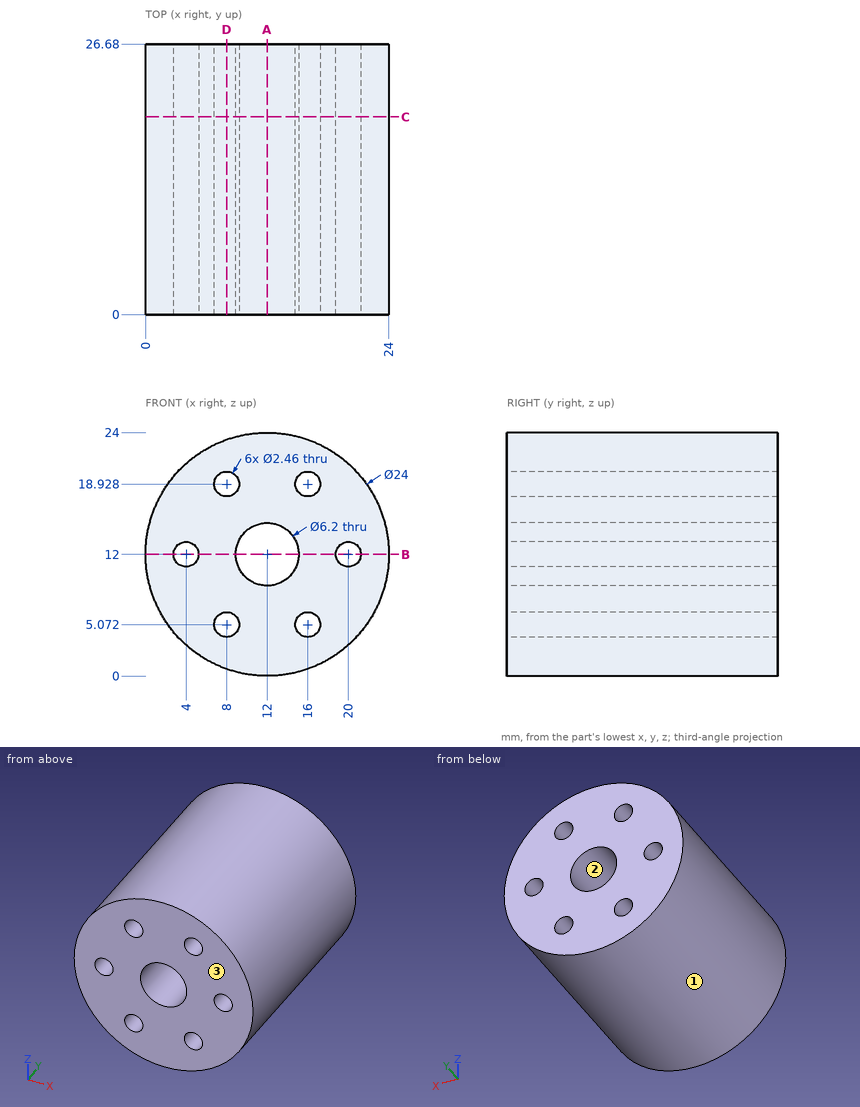
Geometry: see drawing. Coordinates: mm, zero at the bounding-box minimum. Give positions to 0.01 mm unless a question says otherwise; leave off trailing zeros. Order: outer loops, then holes, each group sorted by start corner. A loop starts at its lowest first (then second) coordinate and runs counter-clockwise, first axis right, second up. Notation, with made-up numbers: (77, -11.75) -> (99, -11.75) arc R14 cw to (99, -1.75) -> close; hole circle Ø9 at (-37.5, 75). An arc over 180 degrees is marked (long way). Write each question's results on one line, items separated by ' | '.
1) Cut plane D-D (x = 8). Output: boundary loops of the cut face in (y, z).
Geometry says:
outline: (0, 0.69) -> (26.68, 0.69) -> (26.68, 3.84) -> (0, 3.84) -> close; (0, 6.3) -> (26.68, 6.3) -> (26.68, 17.7) -> (0, 17.7) -> close; (0, 20.16) -> (26.68, 20.16) -> (26.68, 23.31) -> (0, 23.31) -> close
2) Cut plane C-C (y = 19.5). Output: boundary loops of the cut face in (x, z), and give its area (3 significant figures).
Geometry says:
outline: circle Ø24 at (12, 12); hole circle Ø2.46 at (4, 12); hole circle Ø2.46 at (8, 5.07); hole circle Ø2.46 at (8, 18.93); hole circle Ø6.2 at (12, 12); hole circle Ø2.46 at (16, 5.07); hole circle Ø2.46 at (16, 18.93); hole circle Ø2.46 at (20, 12) | area: 394 mm²
3) First-contact query: pin 1 Ø12 at (y, z) = (8.5, 10.5) entering from +X; pin 2 Ø2 at (x, z) = (20, 12) entering from -Y; pin 3 Ø2 at (x, y) = (6, 16.5) entering from -Z; pin 4 Ø10 at (y, z) = (12.5, 21.5) entering from +X. Flat tips, straight axial feed; report the tip coordinate or a pass-through.
Geometry says:
pin 1: stops at x = 24 | pin 2: passes through | pin 3: stops at z = 1.09 | pin 4: stops at x = 23.12
4) Draft query along X for the marked faces 1, 2 and 3. Return one class per face: released by +X, released by -X, zero draft, split by the parting line, or undercut.
Geometry says:
face 1: split by the parting line | face 2: undercut | face 3: zero draft
5) Cut plane A-A (x = 12). Output: boundary loops of the cut face in (y, z), and give its area (3 significant figures).
Geometry says:
outline: (0, 0) -> (26.68, 0) -> (26.68, 8.9) -> (0, 8.9) -> close; (0, 15.1) -> (26.68, 15.1) -> (26.68, 24) -> (0, 24) -> close | area: 475 mm²
6) Line query: line 1 along Z through (x, y) = (8, 21); line 2 along X through (y, z) = (17, 13) (1 decimal); line 3 along Z through (x, y) = (12, 17.25). Output: solid intervals per line, ascending.
Geometry says:
line 1: z = 0.69 to 3.84, 6.3 to 17.7, 20.16 to 23.31 | line 2: x = 0 to 3.3, 4.7 to 9.1, 14.9 to 19.3, 20.7 to 24 | line 3: z = 0 to 8.9, 15.1 to 24
7) Cut plane B-B (z = 12). Output: boundary loops of the cut face in (x, y), and give its area (3 significant figures).
Geometry says:
outline: (0, 0) -> (2.77, 0) -> (2.77, 26.68) -> (0, 26.68) -> close; (5.23, 0) -> (8.9, 0) -> (8.9, 26.68) -> (5.23, 26.68) -> close; (15.1, 0) -> (18.77, 0) -> (18.77, 26.68) -> (15.1, 26.68) -> close; (21.23, 0) -> (24, 0) -> (24, 26.68) -> (21.23, 26.68) -> close | area: 344 mm²
